The model under review builds one solid part; all positions refer to its coordinate system, in mm. Round coordinates to 2 decimals unless told otherwise and drop trailing zeros. Write each loop counter-clockwise with the first axis right and the second up, starting at its lowest first coordinate (ties: lowest second). Pieces come first, ordered by that corner, then holes. Notation, with made-up numbers: M 72,2 L 81,2 A20 cw 81,34 Z; hole C 11,79 d10. An arc over 180 degrees is marked long. One line per item, written item: value. Start each with the question number.
1) Take a section at D-D, the plane z = 2.6. State how many separate pieces and enclosed holes the cut face has, and give its area (3 significant figures).
2) Take a section at A-A, the plane x = -143.25. Write out the cut boundary in (y, z).
3) Take a section at B-B, the plane x = -44.85. Write out the cut boundary in (y, z), and give its area (3 significant figures).
4) For P1, Ø4.5, axis at x = -251.15, y = 0.85, coming from the -Z side; P2, Ø2, axis at y = -27, z = 2.5, coming from the +X side, all flat-tipped, find the tip position at first contact; note any pin that passes through.
5) Mouldability with a two-part tool opening along Y and no side actions: class faces 1 (the face through (22.6, 42.9, 2)), 2 (the face through (22.7, -26.6, 2)), 3 (the face through (-117, 9, 0)), 4 (the face through (-91.196, 19.524, 2.028)) as +Y half, -Y half, draft (parallel to the pull), parting line (faces both ways), or undercut.
6) Take a section at C-C, the plane x = -227. Write out the cut boundary in (y, z).
7) Wall thickness on probe 1 along X at (y, z) = (1, 2.45); probe 2 along Y at (x, z) = (-104.6, 2.55); probe 3 along Y at (x, z) = (-218, 3.25): over which ranges is each line inside the solid? List them lowest first.
Autodesk Inventor part; units mm, degrees
ref_plane "YZ Plane" through (0, 0, 0) normal (1, 0, 0) x (0, 1, 0)
ref_plane "XZ Plane" through (0, 0, 0) normal (0, 1, 0) x (-1, 0, 0)
ref_plane "XY Plane" through (0, 0, 0) normal (0, 0, 1) x (1, 0, 0)
sketch "Эскиз1" plane through (0, 0, 0) normal (0, 0, 1) x (1, 0, 0)
  circle A0 centre (20.65, -19.15) radius 1.75
  circle A1 centre (20.65, 0.85) radius 1.75
  circle A2 centre (20.65, 20.85) radius 1.75
  circle A3 centre (-251.15, -19.15) radius 1.75
  circle A4 centre (-251.15, 0.85) radius 1.75
  circle A5 centre (-251.15, 20.85) radius 1.75
  line L0 (-255.45, -29.15) -> (-246.85, -29.15)
  line L1 (-255.65, -29.15) -> (-255.65, 270.85)
  line L2 (25.15, 270.85) -> (25.15, -29.15)
  line L3 (25.15, -29.15) -> (-255.65, -29.15)
  line L4 (-255.65, -29.15) -> (-255.65, 45.35)
  line L5 (-255.65, 45.35) -> (25.15, 45.35)
  line L6 (25.15, 45.35) -> (25.15, -29.15)
  point P0 (25.15, 45.35)
extrude "Выдавливание1" add sketch "Эскиз1" along normal blind 4
sketch "Эскиз4" plane through (0, 0, 4) normal (0, 0, 1) x (1, 0, 0)
  circle A0 centre (-177.15, -2.65) radius 5 construction
  line L0 (-177.15, -2.65) -> (-177.15, -29.15) construction
  line L1 (-255.65, -29.15) -> (25.15, -29.15) construction
  circle A1 centre (-177.15, -4.15) radius 5
  point P0 (0, 0)
  dimension "d30" = 10
  dimension "d31" = 25
extrude "Выдавливание4" cut sketch "Эскиз4" against normal blind 10
sketch "Эскиз5" plane through (0, 0, 4) normal (0, 0, 1) x (1, 0, 0)
  line L0 (-127.9, -12.65) -> (-102.6, -12.65)
  line L1 (-102.6, -12.65) -> (-102.6, 4.35)
  line L2 (-102.6, 4.35) -> (-127.9, 4.35)
  line L3 (-127.9, 4.35) -> (-127.9, -12.65)
  line L4 (-127.9, -12.65) -> (-102.6, 4.35) construction
  line L5 (-102.6, -12.65) -> (-127.9, 4.35) construction
  circle A0 centre (-125.9, -15.9) radius 1.35
  line L6 (-115.25, -4.15) -> (-115.25, 2.5103)
  line L7 (-115.25, -4.15) -> (-117.239, -4.15)
  circle A1 centre (-104.6, -15.9) radius 1.35
  circle A2 centre (-125.9, 7.6) radius 1.35
  circle A3 centre (-104.6, 7.6) radius 1.35
  line L8 (-255.65, -29.15) -> (25.15, -29.15)
  line L9 (-115.25, -29.15) -> (-115.25, -2.4897) construction
  point P0 (0, 0)
  dimension "d33" = 17
  dimension "d39" = 2.7
  dimension "d40" = 3.25
  dimension "d41" = 2
  dimension "d45" = 25.3
  dimension "d46" = 25
extrude "Выдавливание5" cut sketch "Эскиз5" against normal blind 10
sketch "Эскиз6" plane through (0, 0, 4) normal (0, 0, 1) x (1, 0, 0)
  line L0 (-127.9, -12.65) -> (-127.9, 4.35) construction
  line L1 (-101.8454, -4.15) -> (-167.9603, -4.15) construction
  circle A0 centre (-44.85, -4.15) radius 11
  line L2 (-255.65, -29.15) -> (25.15, -29.15)
  circle A1 centre (-87.25, 19.35) radius 3.95
  line L3 (-127.9, 4.35) -> (-102.6, 4.35)
  line L4 (-102.6, 4.35) -> (-102.6, -12.65)
  line L5 (-87.25, 19.35) -> (-143.25, 19.35) construction
  line L6 (-115.25, 4.35) -> (-115.25, 38.684) construction
  circle A2 centre (-103.25, 19.35) radius 3.95
  line L7 (25.15, -29.15) -> (25.15, 45.35)
  circle A3 centre (-123.25, 19.35) radius 5.5
  circle A4 centre (-143.25, 19.35) radius 5.5
  point P0 (0, 0)
  point P1 (-127.9, -4.15)
  point P2 (-115.25, 19.35)
  dimension "d54" = 22
  dimension "d59" = 25
  dimension "d61" = 7.9
  dimension "d62" = 15
  dimension "d67" = 16
  dimension "d72" = 70
  dimension "d79" = 11
  dimension "d80" = 11
  dimension "d81" = 20
  dimension "d82" = 20
extrude "Выдавливание6" cut sketch "Эскиз6" against normal blind 10
chamfer "Фаска1" distance 5 angle 45 4 edges at (25.15, 45.35, 2) (-255.65, 45.35, 2) (-255.65, -29.15, 2) (25.15, -29.15, 2)
sketch "Эскиз7" plane through (0, 0, 4) normal (0, 0, 1) x (1, 0, 0)
  line L0 (-100.85, -29.15) -> (-100.85, -25.15)
  line L1 (-100.85, -25.15) -> (-84.85, -25.15)
  line L2 (-84.85, -25.15) -> (-84.85, -29.15)
  line L3 (-84.85, -29.15) -> (-100.85, -29.15)
  line L4 (-48.85, -29.15) -> (-48.85, -25.15)
  line L5 (-48.85, -25.15) -> (-32.85, -25.15)
  line L6 (-32.85, -25.15) -> (-32.85, -29.15)
  line L7 (-32.85, -29.15) -> (-48.85, -29.15)
  line L8 (19.15, -25.15) -> (19.15, -29.15)
  line L9 (19.15, -29.15) -> (3.15, -29.15)
  line L10 (3.15, -29.15) -> (3.15, -25.15)
  line L11 (3.15, -25.15) -> (19.15, -25.15)
  line L12 (-204.85, -29.15) -> (-204.85, -25.15)
  line L13 (-204.85, -25.15) -> (-188.85, -25.15)
  line L14 (-188.85, -25.15) -> (-188.85, -29.15)
  line L15 (-188.85, -29.15) -> (-204.85, -29.15)
  line L16 (-152.85, -29.15) -> (-152.85, -25.15)
  line L17 (-152.85, -25.15) -> (-136.85, -25.15)
  line L18 (-136.85, -25.15) -> (-136.85, -29.15)
  line L19 (-136.85, -29.15) -> (-152.85, -29.15)
  line L20 (-126.85, -29.15) -> (-126.85, -25.15)
  line L21 (-126.85, -25.15) -> (-110.85, -25.15)
  line L22 (-110.85, -25.15) -> (-110.85, -29.15)
  line L23 (-110.85, -29.15) -> (-126.85, -29.15)
  line L24 (-178.85, -29.15) -> (-178.85, -25.15)
  line L25 (-178.85, -25.15) -> (-162.85, -25.15)
  line L26 (-162.85, -25.15) -> (-162.85, -29.15)
  line L27 (-162.85, -29.15) -> (-178.85, -29.15)
  line L28 (-230.85, -29.15) -> (-230.85, -25.15)
  line L29 (-230.85, -25.15) -> (-214.85, -25.15)
  line L30 (-214.85, -25.15) -> (-214.85, -29.15)
  line L31 (-214.85, -29.15) -> (-230.85, -29.15)
  line L32 (-6.85, -25.15) -> (-6.85, -29.15)
  line L33 (-6.85, -29.15) -> (-22.85, -29.15)
  line L34 (-22.85, -29.15) -> (-22.85, -25.15)
  line L35 (-22.85, -25.15) -> (-6.85, -25.15)
  line L36 (-74.85, -29.15) -> (-74.85, -25.15)
  line L37 (-74.85, -25.15) -> (-58.85, -25.15)
  line L38 (-58.85, -25.15) -> (-58.85, -29.15)
  line L39 (-58.85, -29.15) -> (-74.85, -29.15)
  line L40 (-249.65, -29.15) -> (-249.65, -25.15)
  line L41 (-249.65, -25.15) -> (-236.85, -25.15)
  line L42 (-236.85, -25.15) -> (-236.85, -29.15)
  line L43 (-236.85, -29.15) -> (-249.65, -29.15)
extrude "Выдавливание7" cut sketch "Эскиз7" against normal blind 4
sketch "Эскиз8" plane through (0, 0, 4) normal (0, 0, 1) x (1, 0, 0)
  line L0 (-32.85, -25.15) -> (-48.85, -25.15) construction
  line L1 (-48.85, -25.15) -> (-58.9685, -29.0911) construction
  circle A0 centre (-53.9092, -27.1206) radius 1.65
  line L2 (-162.85, -25.15) -> (-178.85, -25.15) construction
  line L3 (-188.85, -29.15) -> (-178.85, -29.15) construction
  line L4 (-178.85, -25.15) -> (-188.85, -29.15) construction
  circle A1 centre (-183.85, -27.15) radius 1.65
  point P0 (0, 0)
  dimension "d75" = 3.3
  dimension "d76" = 3.3
extrude "Выдавливание8" cut sketch "Эскиз8" against normal blind 4
properties part number "креп_мотора" material "Древесина (береза)"
Checked values:
1. separate pieces: 1
1. enclosed holes: 19
1. area: 18,900 mm2
2. outline: M -25.15,0 L 13.85,0 L 13.85,4 L -25.15,4 Z; M 24.85,0 L 45.35,0 L 45.35,4 L 24.85,4 Z
3. outline: M -25.15,0 L -15.15,0 L -15.15,4 L -25.15,4 Z; M 6.85,0 L 45.35,0 L 45.35,4 L 6.85,4 Z
3. area: 194 mm2
4. P1: stops at z = 0
4. P2: stops at x = 23.3
5. face 1: +Y half
5. face 2: -Y half
5. face 3: draft
5. face 4: undercut
6. outline: M -25.15,0 L 45.35,0 L 45.35,4 L -25.15,4 Z
7. probe 1: x = -255.65 to -252.89, -249.41 to -127.9, -102.6 to -54.57, -35.13 to 18.91, 22.39 to 25.15
7. probe 2: y = -29.15 to -17.25, -14.55 to -12.65, 4.35 to 6.25, 8.95 to 15.64, 23.06 to 45.35
7. probe 3: y = -25.15 to 45.35
